from build123d import *

# Parameters (mm, degrees)
SKETCH1_W                                  = 59
SKETCH1_H                                  = 50
BOSS_EXTRUDE1_DEPTH                        = 10
SKETCH2_R                                  = 2.7
CUT_EXTRUDE1_DEPTH                         = 10
MIRROR1_AT_THE_SECOND_PLANE_COPY_1_SKETC_R = 2.7
MIRROR1_AT_THE_SECOND_PLANE_COPY_1_DEPTH   = 10
SKETCH9_W                                  = 59
SKETCH9_H                                  = 10
BOSS_EXTRUDE10_DEPTH                       = 18.461375068
SKETCH12_W                                 = 59
SKETCH12_H                                 = 20
BOSS_EXTRUDE11_DEPTH                       = 19.770139482
SKETCH13_W                                 = 19.770139482
SKETCH13_H                                 = 20
BOSS_EXTRUDE12_DEPTH                       = 70
SKETCH14_W                                 = 15
SKETCH14_H                                 = 20
BOSS_EXTRUDE13_DEPTH                       = 80
BOSS_EXTRUDE14_DEPTH                       = 20
BOSS_EXTRUDE15_DEPTH                       = 5
SKETCH16_W                                 = 199
SKETCH16_H                                 = 5
CUT_EXTRUDE3_DEPTH                         = 109.350147663


with BuildPart() as part:
    # Sketch1 → Boss-Extrude1 (new body)
    with BuildSketch(Plane.XY):
        Rectangle(SKETCH1_W, SKETCH1_H)
    extrude(amount=BOSS_EXTRUDE1_DEPTH)

    # Sketch2 → Cut-Extrude1 (cut)
    with BuildSketch(Plane.XY.offset(10)):
        with Locations((-20, 15)):
            Circle(SKETCH2_R)
    cut_extrude1 = extrude(amount=-CUT_EXTRUDE1_DEPTH, mode=Mode.SUBTRACT)

    # Mirror1: Cut-Extrude1 across plane
    add(cut_extrude1.mirror(Plane.ZX), mode=Mode.SUBTRACT)

    # Mirror1 at the second plane: Cut-Extrude1 across plane
    add(cut_extrude1.mirror(Plane(origin=(0, 0, 0), x_dir=(0, 0, 1), z_dir=(1, 0, 0))), mode=Mode.SUBTRACT)

    # Mirror1 at the second plane copy 1 sketc → Mirror1 at the second plane copy 1 (cut)
    with BuildSketch(Plane(origin=(0, 0, 10), x_dir=(-1, 0, 0), z_dir=(0, 0, 1))):
        with Locations((-20, 15)):
            Circle(MIRROR1_AT_THE_SECOND_PLANE_COPY_1_SKETC_R)
    extrude(amount=-MIRROR1_AT_THE_SECOND_PLANE_COPY_1_DEPTH, mode=Mode.SUBTRACT)

    # Sketch9 → Boss-Extrude10 (add)
    with BuildSketch(Plane(origin=(0, 25, 0), x_dir=(1, 0, 0), z_dir=(0, 1, 0))):
        with Locations((0, -5)):
            Rectangle(SKETCH9_W, SKETCH9_H)
    extrude(amount=BOSS_EXTRUDE10_DEPTH)

    # Sketch12 → Boss-Extrude11 (add)
    with BuildSketch(Plane(origin=(0, 0, 0), x_dir=(-1, 0, 0), z_dir=(0, 0, -1))):
        with Locations((0, 33.461375068)):
            Rectangle(SKETCH12_W, SKETCH12_H)
    extrude(amount=BOSS_EXTRUDE11_DEPTH)

    # Sketch13 → Boss-Extrude12 (add)
    with BuildSketch(Plane.ZY.offset(29.5)):
        with Locations((-9.885069741, 33.461375068)):
            Rectangle(SKETCH13_W, SKETCH13_H)
    boss_extrude12 = extrude(amount=BOSS_EXTRUDE12_DEPTH)

    # Sketch14 → Boss-Extrude13 (add)
    with BuildSketch(Plane(origin=(0, 0, -19.770139482), x_dir=(-1, 0, 0), z_dir=(0, 0, -1))):
        with Locations((92, 33.461375068)):
            Rectangle(SKETCH14_W, SKETCH14_H)
    boss_extrude13 = extrude(amount=BOSS_EXTRUDE13_DEPTH)

    # Mirror2: Boss-Extrude12, Boss-Extrude13 across plane
    add(boss_extrude12.mirror(Plane(origin=(0, 0, 0), x_dir=(0, 0, 1), z_dir=(1, 0, 0))))
    add(boss_extrude13.mirror(Plane(origin=(0, 0, 0), x_dir=(0, 0, 1), z_dir=(1, 0, 0))))

    # Sketch15 → Boss-Extrude14 (add)
    with BuildSketch(Plane(origin=(0, 43.461375068, 0), x_dir=(1, 0, 0), z_dir=(0, 1, 0))):
        Polygon((-84.5, 19.770139482), (-54.5, 19.770139482), (-84.5, 49.770139482), align=None)
    boss_extrude14 = extrude(amount=-BOSS_EXTRUDE14_DEPTH)

    # Mirror3: Boss-Extrude14 across plane
    add(boss_extrude14.mirror(Plane(origin=(0, 0, 0), x_dir=(0, 0, 1), z_dir=(1, 0, 0))))

    # Sketch19 → Boss-Extrude15 (add)
    with BuildSketch(Plane(origin=(10, 0, 0), x_dir=(0, 0, -1), z_dir=(1, 0, 0))):
        Polygon((0, -25), (19.770139482, 23.461375068), (0, 23.461375068), align=None)
    boss_extrude15 = extrude(amount=-BOSS_EXTRUDE15_DEPTH)

    # Mirror4: Boss-Extrude15 across plane
    add(boss_extrude15.mirror(Plane(origin=(0, 0, 0), x_dir=(0, 0, 1), z_dir=(1, 0, 0))))

    # Sketch16 → Cut-Extrude3 (cut)
    with BuildSketch(Plane.XY.offset(-120)):
        with Locations((0, 33.461375068)):
            Rectangle(SKETCH16_W, SKETCH16_H)
    extrude(amount=CUT_EXTRUDE3_DEPTH, mode=Mode.SUBTRACT)


solid = part.part
Input: part model. Units: mm. Frame: model coordinates. A direction names the side the tool comes from. Coordinates: 2 decimals unless noted, no trailing zeros. Order: outer loops, then holes, each group sorted by start corner. A loop starts at its lowest first (then second) coordinate and runs counter-clockwise, first axis right, second up.
1. Cut plane A-A, the plane x = -20. Return loops of the section in (y, z).
Checked values:
outline: (-25, 0) - (-17.7, 0) - (-17.7, 10) - (-25, 10) - close; (-12.3, 0) - (12.3, 0) - (12.3, 10) - (-12.3, 10) - close; (17.7, 0) - (23.46, 0) - (23.46, -19.77) - (30.96, -19.77) - (30.96, -10.65) - (35.96, -10.65) - (35.96, -19.77) - (43.46, -19.77) - (43.46, 10) - (17.7, 10) - close
2. Draft query along Y for faces 5 (the flat face through (-71, 23.461, -28)), 6 (the flat face through (-64, 33, 0)), 7 (the cylindrical face through (-18.548, -17.277, 5.07)). Return one class per face: +Y half, -Y half, draft (parallel to the pull), parting line (faces both ways), or undercut.
Checked values:
face 5: -Y half
face 6: draft
face 7: undercut
3. Cut plane B-B, the plane z = -38. Return loops of the section in (x, y).
Checked values:
outline: (-99.5, 23.46) - (-72.73, 23.46) - (-72.73, 30.96) - (-99.5, 30.96) - close; (-99.5, 35.96) - (-72.73, 35.96) - (-72.73, 43.46) - (-99.5, 43.46) - close; (72.73, 23.46) - (99.5, 23.46) - (99.5, 30.96) - (72.73, 30.96) - close; (72.73, 35.96) - (99.5, 35.96) - (99.5, 43.46) - (72.73, 43.46) - close
4. Access query for faces 1 (the flat face through (-29.5, 9, 5)), 2 (the flat face through (64, 33, 0)), 3 (the flat face through (-5, 5, -8)), 4 (the flat face through (-69.29, 27.26, -34.56)). Directions: +Z, -Z, +X, -X, +Y, -Y. A direction counts if a zero-diameter tool reaches every point of the face in a straight line with its end or side. Return the directions, or none.
Checked values:
face 1: +Z, -X, +Y, -Y
face 2: +Z, +X, +Y, -Y
face 3: -Z, -Y
face 4: -Z, +Y, -Y
5. Cut plane C-C, the plane y = -15. Return loops of the section in (x, z), plus the area to 3 significant figures.
Checked values:
outline: (-29.5, 0) - (-22.7, 0) - (-22.7, 10) - (-29.5, 10) - close; (-17.3, 0) - (-10, 0) - (-10, -4.08) - (-5, -4.08) - (-5, 0) - (5, 0) - (5, -4.08) - (10, -4.08) - (10, 0) - (17.3, 0) - (17.3, 10) - (-17.3, 10) - close; (22.7, 0) - (29.5, 0) - (29.5, 10) - (22.7, 10) - close
area: 523 mm2
6. Cut plane D-D, the plane x = -45. Return loops of the section in (y, z).
Checked values:
outline: (23.46, -19.77) - (30.96, -19.77) - (30.96, -10.65) - (35.96, -10.65) - (35.96, -19.77) - (43.46, -19.77) - (43.46, 0) - (23.46, 0) - close
7. Contact query for flat-ended pins moving along their axis: P1, Ø4, axis at x = 4.5, y = 28, coming from the -Z side; P2, Ø10, axis at x = -18, y = -0.5, coming from the -Z side; P3, Ø5, axis at y = 11.5, z = 6.5, coming from the -X side. Output: stop coordinate, or through.
Checked values:
P1: stops at z = -19.77
P2: stops at z = 0
P3: stops at x = -29.5
8. Ray query, line 1 along X through (y, z) = (-15, 5); line 2 along Y through (x, z) = (20, 7); line 3 along Y through (x, z) = (91.5, -39.5). Return the intervals inside material, ascending.
Checked values:
line 1: x = -29.5 to -22.7, -17.3 to 17.3, 22.7 to 29.5
line 2: y = -25 to -17.7, -12.3 to 12.3, 17.7 to 43.46
line 3: y = 23.46 to 30.96, 35.96 to 43.46
